from build123d import *

# Parameters (mm, degrees)
SKETCH_1_R          = 11
SKETCH_1_R_2        = 1.5
EXTRUDE_1_DEPTH     = 2
EXTRUDE_2_DEPTH     = 3
FILLET_1_R          = 2
FILLET_2_R          = 2
FILLET_3_R          = 2
CHAMFER_1_SIZE      = 0.3
SKETCH_3_R          = 1.6
CUT_EXTRUDE_1_DEPTH = 3


with BuildPart() as part:
    # 草图1 → 凸台-拉伸1 (new body)
    with BuildSketch(Plane(origin=(0, 0, 0), x_dir=(1, 0, 0), z_dir=(0, 1, 0))):
        Polygon((16.8, 21), (-16.8, 21), (-21, 16.8), (-21, -16.8), (-16.8, -21), (16.8, -21), (21, -16.8), (21, 16.8), align=None)
        with Locations(Location((0, 0, 0), (0, 0, 270))):
            Circle(SKETCH_1_R, mode=Mode.SUBTRACT)
        with Locations(Location((-15.5, 15.5, 0), (0, 0, 270))):
            Circle(SKETCH_1_R_2, mode=Mode.SUBTRACT)
        with Locations(Location((15.5, 15.5, 0), (0, 0, 90))):
            Circle(SKETCH_1_R_2, mode=Mode.SUBTRACT)
        with Locations(Location((15.5, -15.5, 0), (0, 0, 270))):
            Circle(SKETCH_1_R_2, mode=Mode.SUBTRACT)
        with Locations(Location((-15.5, -15.5, 0), (0, 0, 90))):
            Circle(SKETCH_1_R_2, mode=Mode.SUBTRACT)
    extrude(amount=EXTRUDE_1_DEPTH)

    # 草图2 → 凸台-拉伸2 (add)
    with BuildSketch(Plane.XY.offset(21)):
        Polygon((-21, -70), (21, -70), (21, -4.2), (16.8, 0), (16.8, 2), (-16.8, 2), (-16.8, 0), (-21, -4.2), align=None)
    extrude(amount=EXTRUDE_2_DEPTH)

    # 圆角1
    fillet_1_edges = [part.edges().sort_by_distance(p)[0] for p in [
        (0, 2, 24),
    ]]
    fillet(fillet_1_edges, radius=FILLET_1_R)

    # 圆角2
    fillet_2_edges = [part.edges().sort_by_distance(p)[0] for p in [
        (-21, -70, 22.5),
        (21, -70, 22.5),
    ]]
    fillet(fillet_2_edges, radius=FILLET_2_R)

    # 圆角3
    fillet_3_edges = [part.edges().sort_by_distance(p)[0] for p in [
        (21, 1, -16.8),
        (21, 1, 16.8),
        (-21, 1, 16.8),
        (-21, 1, -16.8),
        (-16.8, 1, -21),
        (16.8, 1, -21),
        (-21, -4.2, 22.5),
        (21, -4.2, 22.5),
    ]]
    fillet(fillet_3_edges, radius=FILLET_3_R)

    # 倒角1
    # the kernel refuses this chamfer: 0.3 mm, written as the material it takes off along each edge
    with BuildSketch(Plane(origin=(20.414213562, -3.614213562, 24), x_dir=(-0.7068394360706586, -0.7068394360706884, 0.027495876610584332), z_dir=(-0.7071067811865624, 0.7071067811865326, 0))) as chamfer_1_piece_1_section:
        Polygon((CHAMFER_1_SIZE * 0.999621916911, -CHAMFER_1_SIZE * 0.0274958766106), (-CHAMFER_1_SIZE * 0.0274958766106, -CHAMFER_1_SIZE * 0.999621916911), (0, 0), align=None)
    chamfer_1_piece_1 = extrude(amount=5.882774734, mode=Mode.PRIVATE)
    chamfer_1_piece_1 = split(chamfer_1_piece_1, bisect_by=Plane(origin=(16.8, -3.46784849, 23.913969067), z_dir=(1, 0, 0)), keep=Keep.TOP, mode=Mode.PRIVATE)
    add(chamfer_1_piece_1, mode=Mode.SUBTRACT)
    with BuildSketch(Plane(origin=(20.414213562, -3.614213562, 24), x_dir=(-0.7068394360706586, -0.7068394360706884, 0.027495876610584332), z_dir=(-0.7071067811865624, 0.7071067811865326, 0))) as chamfer_1_piece_2_section:
        Polygon((CHAMFER_1_SIZE * 0.999621916911, -CHAMFER_1_SIZE * 0.0274958766106), (-CHAMFER_1_SIZE * 0.0274958766106, -CHAMFER_1_SIZE * 0.999621916911), (0, 0), align=None)
    chamfer_1_piece_2 = extrude(amount=5.882774734, mode=Mode.PRIVATE)
    chamfer_1_piece_2 = chamfer_1_piece_2 - Plane(origin=(16.713155259, 0, 22), x_dir=(0, 1, 0), z_dir=(-1, 0, 0)) * Cylinder(2, 13, mode=Mode.PRIVATE)
    add(chamfer_1_piece_2, mode=Mode.SUBTRACT)
    with BuildSketch(Plane(origin=(-21, -5.028427125, 24), x_dir=(0.9996219169112968, 0, 0.027495876610584464), z_dir=(0, -1, 0)), Plane(origin=(21, -68, 24), x_dir=(-0.9996219169112968, 0, 0.027495876610584464), z_dir=(0, 1, 0))) as chamfer_1_piece_3:
        Polygon((CHAMFER_1_SIZE * 0.999621916911, -CHAMFER_1_SIZE * 0.0274958766106), (-CHAMFER_1_SIZE * 0.0274958766106, -CHAMFER_1_SIZE * 0.999621916911), (0, 0), align=None)
    extrude(amount=62.971572875, mode=Mode.SUBTRACT)
    with BuildSketch(Plane(origin=(-19, -5.028427125, 24), x_dir=(-0.7071067811865533, 0.7071067811865418, 0), z_dir=(0.7071067811865418, 0.7071067811865533, 0))) as chamfer_1_piece_4:
        Polygon((2 - CHAMFER_1_SIZE, 0), (2, -CHAMFER_1_SIZE), (2, 0), align=None)
    revolve(axis=Axis((-19, -5.028427125, 24), (0, 0, 1)), revolution_arc=45, mode=Mode.SUBTRACT)
    with BuildSketch(Plane(origin=(19, -5.028427125, 24), x_dir=(1, 0, 0), z_dir=(0, -1, 0))) as chamfer_1_piece_5:
        Polygon((2 - CHAMFER_1_SIZE, 0), (2, -CHAMFER_1_SIZE), (2, 0), align=None)
    revolve(axis=Axis((19, -5.028427125, 24), (0, 0, 1)), revolution_arc=45, mode=Mode.SUBTRACT)
    with BuildSketch(Plane(origin=(-16.254463656, 0.545536344, 24), x_dir=(0.7068394360706796, -0.7068394360706673, 0.027495876610584523), z_dir=(-0.7071067811865415, -0.7071067811865537, 0))) as chamfer_1_piece_6_section:
        Polygon((CHAMFER_1_SIZE * 0.999621916911, -CHAMFER_1_SIZE * 0.0274958766106), (-CHAMFER_1_SIZE * 0.0274958766106, -CHAMFER_1_SIZE * 0.999621916911), (0, 0), align=None)
    chamfer_1_piece_6 = extrude(amount=5.882774734, mode=Mode.PRIVATE)
    chamfer_1_piece_6 = split(chamfer_1_piece_6, bisect_by=Plane(origin=(-16.8, -0.406139504, 23.857619538), z_dir=(-1, 0, 0)), keep=Keep.TOP, mode=Mode.PRIVATE)
    add(chamfer_1_piece_6, mode=Mode.SUBTRACT)
    with BuildSketch(Plane(origin=(-16.254463656, 0.545536344, 24), x_dir=(0.7068394360706796, -0.7068394360706673, 0.027495876610584523), z_dir=(-0.7071067811865415, -0.7071067811865537, 0))) as chamfer_1_piece_7_section:
        Polygon((CHAMFER_1_SIZE * 0.999621916911, -CHAMFER_1_SIZE * 0.0274958766106), (-CHAMFER_1_SIZE * 0.0274958766106, -CHAMFER_1_SIZE * 0.999621916911), (0, 0), align=None)
    chamfer_1_piece_7 = extrude(amount=5.882774734, mode=Mode.PRIVATE)
    chamfer_1_piece_7 = chamfer_1_piece_7 - Plane(origin=(-16.713155259, 0, 22), x_dir=(0, 1, 0), z_dir=(-1, 0, 0)) * Cylinder(2, 13, mode=Mode.PRIVATE)
    add(chamfer_1_piece_7, mode=Mode.SUBTRACT)
    with BuildSketch(Plane(origin=(-19, -70, 24), x_dir=(0, 0.9996219169112968, 0.0274958766105851), z_dir=(1, 0, 0))) as chamfer_1_piece_8:
        Polygon((CHAMFER_1_SIZE * 0.999621916911, -CHAMFER_1_SIZE * 0.0274958766106), (-CHAMFER_1_SIZE * 0.0274958766106, -CHAMFER_1_SIZE * 0.999621916911), (0, 0), align=None)
    extrude(amount=38, mode=Mode.SUBTRACT)
    with BuildSketch(Plane(origin=(19, -68, 24), x_dir=(1, 0, 0), z_dir=(0, 1, 0))) as chamfer_1_piece_9:
        Polygon((2 - CHAMFER_1_SIZE, 0), (2, CHAMFER_1_SIZE), (2, 0), align=None)
    revolve(axis=Axis((19, -68, 24), (0, 0, -1)), revolution_arc=90, mode=Mode.SUBTRACT)
    with BuildSketch(Plane(origin=(-19, -68, 24), x_dir=(-1, 0, 0), z_dir=(0, 1, 0))) as chamfer_1_piece_10:
        Polygon((2 - CHAMFER_1_SIZE, 0), (2, -CHAMFER_1_SIZE), (2, 0), align=None)
    revolve(axis=Axis((-19, -68, 24), (0, 0, 1)), revolution_arc=90, mode=Mode.SUBTRACT)

    # 草图3 → 切除-拉伸1 (cut)
    with BuildSketch(Plane(origin=(0, 0, 21), x_dir=(-1, 0, 0), z_dir=(0, 0, -1))):
        with Locations((-16, -65)):
            Circle(SKETCH_3_R)
        with Locations((16, -65)):
            Circle(SKETCH_3_R)
    extrude(amount=-CUT_EXTRUDE_1_DEPTH, mode=Mode.SUBTRACT)


solid = part.part
Input: part model. Units: mm. Frame: model coordinates. A direction names the side the tool comes from. Coordinates: 2 decimals unless noted, no trailing zeros. Write each loop counter-clockwise with the first axis right and the second up, starting at its lowest first coordinate (ties: lowest second). Pieces come first, ordered by that corner, then holes. Notation, with made-up numbers: M -29.75,-19 L 22.25,-19 A18 cw 22.25,-6 Z; hole C 14.25,-10 d1. An arc over 180 degrees is marked long. Answer as a JSON object with one key per item and string values. Group by question number.
(1) Section A-A on y = -65. Output: boundary loops of the cut face in (x, z), plus the area to 3 significant figures.
(2) Section B-B on x = 5.5. Output: boundary loops of the cut face in (y, z), plus the area to 3 significant figures.
(3) Ray query, line 1 along X through (y, z) = (0.6, 15.5); line 2 along X through (y, z) = (1, 15); line 3 along Z through (x, y) = (-15.5, -22.5). Return the intervals inside material, ascending. Write a range as [from, to].
(4) Section C-C on z = 0. Output: boundary loops of the cut face in (x, y).
(5) Contact query for flat-ended pins moving along their axis: P1, Ø3, axis at x = 16, y = -65, coming from the -Z side; P2, Ø3.5, axis at x = 15.5, z = 15.5, coming from the -Y side; P3, Ø21, axis at x = 2.5, y = -34.5, coming from the -Z side; P4, Ø2.5, axis at y = 0.5, z = 22, coming from the -X side. Output: stop coordinate, or through.
(6) Set-up query: faces 5 (the face through (16.8, 1, 22)), 6 (the face through (21, 1, 0)). Return all of +Z, -Z, +X, -X, +Y, -Y with unobstructed straight access to the full face (end or side cutting, diameter ignored); none if empty.
(7) Mould query, pull axis X, two halves, no side actions, for faces 1 (the face through (21, -37, 22)), 2 (the face through (-15.43, 0.99, -17)), 3 (the face through (-15.792, -63.414, 22.479)), 4 (the face through (-9, 2, -9)). Classes: pulls with the +X half, pulls with the -X half, needs draft (parallel to the pull), parting line crosses it, or undercut.
(8) Section D-D on y = -50.5. Output: boundary loops of the cut face in (x, z).
Result set:
{
 "1": {"outline": "M -21,21 L -17.6,21 L -17.6,24 L -20.7,24 L -21,23.7 Z; M -14.4,21 L 14.4,21 L 14.4,24 L -14.4,24 Z; M 17.6,21 L 21,21 L 21,23.7 L 20.7,24 L 17.6,24 Z", "area": "107 mm2"},
 "2": {"outline": "M -70,21 L 0,21 L 0,9.53 L 2,9.53 L 2,22 A2 ccw 0,24 L -69.7,24 L -70,23.7 Z; M 0,-21 L 2,-21 L 2,-9.53 L 0,-9.53 Z", "area": "261 mm2"},
 "3": {"line 1": "x = [-21, -17], [-14, 14], [17, 21]", "line 2": "x = [-21, -16.91], [-14.09, 14.09], [16.91, 21]", "line 3": "z = [21, 24]"},
 "4": {"outline": "M -21,0 L -11,0 L -11,2 L -21,2 Z; M 11,0 L 21,0 L 21,2 L 11,2 Z"},
 "5": {"P1": "passes through", "P2": "stops at y = 0", "P3": "stops at z = 21", "P4": "stops at x = -17.55"},
 "6": {"face 5": "+Z, +X, +Y", "face 6": "+Z, -Z, +X, +Y, -Y"},
 "7": {"face 1": "pulls with the +X half", "face 2": "undercut", "face 3": "undercut", "face 4": "needs draft"},
 "8": {"outline": "M -21,21 L 21,21 L 21,23.7 L 20.7,24 L -20.7,24 L -21,23.7 Z"}
}
